Here's how the part is built. I have some questions about the finished solid (model axes, mm). Round coordinates to 2 decimals unless told otherwise and drop trailing zeros. Write each loop counter-clockwise with the first axis right and the second up, starting at its lowest first coordinate (ties: lowest second). Pieces come first, ordered by that corner, then holes. Notation, with made-up numbers: (89, 24) - (104, 24) arc R10 cw to (104, 30) - close; hole circle Ø10 at (68, 33.5). An arc over 180 degrees is marked (long way). One line per item, written item: value. Start each with the question number.
Item 1: Imagine slicing it at A-A, the plane x = 126. Please give me the cut outline in (y, z).
Item 2: If I drill on line 1 (Y direction, x = 4.5, z = -35.75); line 2 (Z direction, x = 15, y = -7.5); line 3 (Z direction, x = 91, y = -3.5), over which ranges is the centre line in solid material (lowest first)?
Item 3: Thinking about a two-plate mould opening in Z: for faces 1 (the face through (13.98, -0.02, 71.05)), 2 (the face through (185.649, 35, 1)), which applies, released by +Z, released by -Z, zero draft, split by the parting line, or undercut?
Item 4: For P1, Ø4.5, axis at y = -71.11, z = -7.47, coming from the -X side; P2, Ø4, axis at x = 62, y = -23, coming from the +Z side; P3, Ø8, axis at x = 114.5, y = 28, coming from the +Z side; P4, Ø6, axis at y = -29.08, z = 65.32, coming from the -X side, each with a flat end and sliding along its axis, tell me the tip position at first contact or that it passes through.
```python
from build123d import *

# Parameters (mm, degrees)
CIRPATTERN1_COUNT = 15


with BuildPart() as part:
    # Model → Revolve1 (revolve)
    with BuildSketch(Plane.XY, mode=Mode.PRIVATE) as revolve1_sk:
        with BuildLine():
            Line((0, 55.140272), (23.150958, 55.140272))
            ThreePointArc((23.150958, 55.140272), (60.421138671, 50.233559208), (95.151418, 35.847806))
            Line((95.151418, 35.847806), (128.566947896, 16.55534082))
            ThreePointArc((128.566947896, 16.55534082), (133.553991718, 14.489639839), (138.905748896, 13.78506782))
            ThreePointArc((138.905748896, 13.78506782), (139.768990342, 13.856305516), (140.608875713, 14.068091181))
            add(Edge.make_bspline(
                [(140.608875713, 14.068091181), (181.460140896, 28.03089782), (185.649173896, 29.31027082)],
                knots=[0, 0, 0, 1, 1, 1], degree=2))
            Line((185.649173896, 29.31027082), (185.649173896, 80.540272))
            Line((185.649173896, 80.540272), (0, 80.540272))
            Line((0, 80.540272), (0, 55.140272))
        make_face()
    revolve(revolve1_sk.sketch.rotate(Axis((0, 0, 0), (1, 0, 0)), 90), axis=Axis((0, 0, 0), (1, 0, 0)))

    # Sketch3 → 13/64 (0.20313) Diameter Hole1 (revolve, cut)
    with BuildSketch(Plane(origin=(0, 0, 71.5), x_dir=(0, 0, 1), z_dir=(0, 1, 0))):
        Polygon((0, 0), (0, 14.250070783), (2.579751, 12.7), (2.579751, 0), align=None)
    f_13_64_0_20313_diameter_hole1 = revolve(axis=Axis((-6.35, 0, 71.5), (1, 0, 0)), mode=Mode.SUBTRACT)

    # CirPattern1: 13/64 (0.20313) Diameter Hole1 ×15 about axis
    cirpattern1_axis = Axis((0, 0, 0), (1, 0, 0))
    for i in range(1, CIRPATTERN1_COUNT):
        add(f_13_64_0_20313_diameter_hole1.rotate(cirpattern1_axis, i * 360 / CIRPATTERN1_COUNT), mode=Mode.SUBTRACT)


solid = part.part
```
Values follow:
1. outline: circle Ø161.08 at (0, 0); hole circle Ø36.07 at (0, 0)
2. line 1: y = -72.17 to -64.5, -59.34 to -41.98, 41.98 to 59.34, 64.5 to 72.17
2. line 2: z = -80.19 to -54.63, 54.63 to 80.19
2. line 3: z = -80.46 to -37.99, 37.99 to 80.46
3. face 1: undercut
3. face 2: zero draft
4. P1: stops at x = 12.9
4. P2: stops at z = 77.75
4. P3: stops at z = 76.88
4. P4: stops at x = 0
